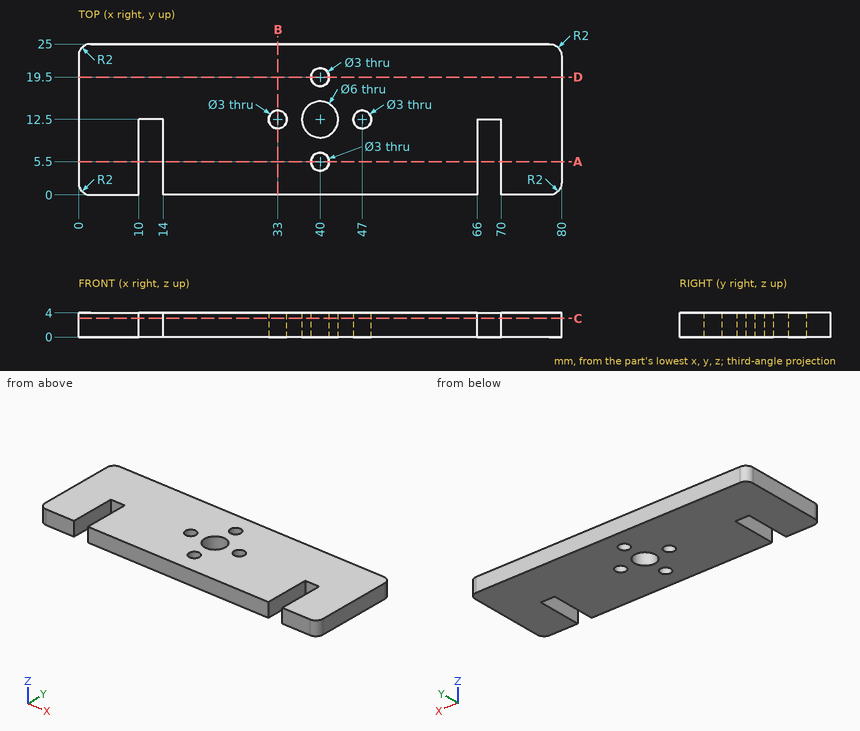
Could you check a few things on this drawing? It's one solid part, dimensions in mm from its lowest x, y, z. Give positions to 0.01 mm unless a question says otherwise; leave off trailing zeros. Order: outer loops, then holes, each group sorted by start corner. A loop starts at its lowest first (then second) coordinate and runs counter-clockwise, first axis right, second up. Notation, with made-up numbers: (-24, 13.25) -> (11, 13.25) arc R21 ccw to (11, 50.25) -> close; hole circle Ø4 at (-16.75, -31.5). An arc over 180 degrees is marked (long way). Answer in a Markdown table with one row per item. Add a question column.
Item 1: Imagine slicing it at C-C (z = 3.1). List the corners of the cut face in (x, y) for me.
Item 2: Imagine slicing it at B-B (x = 33). List the corners of the cut face in (y, z) for me.
Item 3: Imagine slicing it at D-D (y = 19.5). List the corners of the cut face in (x, z) for me.
Item 4: Imagine slicing it at A-A (y = 5.5). List the corners of the cut face in (x, z) for me.
Item 5: I'm going to push flat-ended pins straight in: P1, Ø1.8, axis at x = 33, y = 12.5, coming from the +Z side; P2, Ø1.2, axis at x = 12.5, z = 1, coming from the -Y side. Where does each tip first touch, or does it pass through?
Item 6: Please list where these lines run through material, in increasing order: probe 1 along Y at (x, z) = (40, 2.8); probe 2 along X at (y, z) = (5.5, 1.65); probe 3 along X at (y, z) = (2.75, 2.5).
Result:
| question | item | result |
|---|---|---|
| 1 | outline | (0, 2) arc R2 ccw to (2, 0) -> (10, 0) -> (10, 12.5) -> (14, 12.5) -> (14, 0) -> (66, 0) -> (66, 12.5) -> (70, 12.5) -> (70, 0) -> (78, 0) arc R2 ccw to (80, 2) -> (80, 23) arc R2 ccw to (78, 25) -> (2, 25) arc R2 ccw to (0, 23) -> close; hole circle Ø3 at (33, 12.5); hole circle Ø6 at (40, 12.5); hole circle Ø3 at (40, 5.5); hole circle Ø3 at (40, 19.5); hole circle Ø3 at (47, 12.5) |
| 2 | outline | (0, 0) -> (11, 0) -> (11, 4) -> (0, 4) -> close; (14, 0) -> (25, 0) -> (25, 4) -> (14, 4) -> close |
| 3 | outline | (0, 0) -> (38.5, 0) -> (38.5, 4) -> (0, 4) -> close; (41.5, 0) -> (80, 0) -> (80, 4) -> (41.5, 4) -> close |
| 4 | outline | (0, 0) -> (10, 0) -> (10, 4) -> (0, 4) -> close; (14, 0) -> (38.5, 0) -> (38.5, 4) -> (14, 4) -> close; (41.5, 0) -> (66, 0) -> (66, 4) -> (41.5, 4) -> close; (70, 0) -> (80, 0) -> (80, 4) -> (70, 4) -> close |
| 5 | P1 | through |
| 5 | P2 | y = 12.5 |
| 6 | probe 1 | 0 to 4, 7 to 9.5, 15.5 to 18, 21 to 25 |
| 6 | probe 2 | 0 to 10, 14 to 38.5, 41.5 to 66, 70 to 80 |
| 6 | probe 3 | 0 to 10, 14 to 66, 70 to 80 |
